Here's how the part is built. I have some questions about the finished solid (model axes, mm). Coordinates: 2 decimals unless noted, no trailing zeros. Write each loop counter-clockwise with the first axis right and the second up, starting at its lowest first coordinate (ties: lowest second). Pieces come first, ordered by that corner, then holes.
(1) Imagine slicing it at B-B, the plane y = 0.4. State how many separate pieces and enclosed holes the cut face has, plus the area to 3 significant figures.
(2) Imagine slicing it at A-A, the plane z = 63.56. List the corners of the cut face in (x, y) for me.
(3) For pin 1 Ø1 at (x, y) = (36, 0.5) entering from -Z, with a flat end and sliding along its axis, tell me the tip position at first contact or that it passes through.
(4) Imagine slicing it at C-C, the plane x = 66.72. List the corners of the cut face in (y, z) for me (3 decimals), plus the area to 3 significant figures.
(5) Imagine slicing it at D-D, the plane x = 52.22. List the corners of the cut face in (y, z) for me, plus the area to 3 significant figures.
(6) Thinking about a two-plate mould opening in Z: for faces 1 (the flat face through (-3, 1, 48)), 2 (the cylindrical face through (64.963, 0.986, 68.005)), 3 (the cylindrical face through (76.17, 0.99, 72.1)), which applies, released by +Z, released by -Z, zero draft, split by the parting line, or undercut?
(7) Please list where these lines run through material, in increasing order: probe 1 along X at (y, z) = (1.3, 31.49); probe 2 along Z at (x, y) = (23.5, 1.15); probe 3 along Z at (x, y) = (24, 1.4).
```python
from build123d import *

# Parameters (mm, degrees)
CROQUIS1_R              = 1.8
CROQUIS1_R_2            = 1.5
SALIENTE_EXTRUIR1_DEPTH = 2


with BuildPart() as part:
    # Croquis1 → Saliente-Extruir1 (new body)
    with BuildSketch(Plane(origin=(0, 0, 0), x_dir=(1, 0, 0), z_dir=(0, 1, 0))):
        with BuildLine():
            Line((0.952532669, 2.844763877), (74.672532669, -21.839431846))
            ThreePointArc((74.672532669, -21.839431846), (76.154912525, -22.931711487), (76.72, -24.684195722))
            Line((76.72, -24.684195722), (76.72, -70.365804278))
            ThreePointArc((76.72, -70.365804278), (76.154912525, -72.118288513), (74.672532669, -73.210568154))
            Line((74.672532669, -73.210568154), (0.952532669, -97.894763877))
            ThreePointArc((0.952532669, -97.894763877), (-1.752484236, -97.484912525), (-3, -95.05))
            Line((-3, -95.05), (-3, 0))
            ThreePointArc((-3, 0), (-1.752484236, 2.434912525), (0.952532669, 2.844763877))
        make_face()
        with Locations(Location((25, -26.675, 0), (0, 0, 270))):
            Circle(CROQUIS1_R, mode=Mode.SUBTRACT)
        with Locations(Location((25, -68.395, 0), (0, 0, 270))):
            Circle(CROQUIS1_R, mode=Mode.SUBTRACT)
        with Locations(Location((66.72, -26.675, 0), (0, 0, 270))):
            Circle(CROQUIS1_R, mode=Mode.SUBTRACT)
        with Locations(Location((66.72, -68.395, 0), (0, 0, 270))):
            Circle(CROQUIS1_R, mode=Mode.SUBTRACT)
        with Locations(Location((0, 0, 0), (0, 0, 270))):
            Circle(CROQUIS1_R_2, mode=Mode.SUBTRACT)
        with Locations(Location((0, -95.05, 0), (0, 0, 270))):
            Circle(CROQUIS1_R_2, mode=Mode.SUBTRACT)
        with Locations(Location((52.22, -31.49, 0), (0, 0, 270))):
            Circle(CROQUIS1_R_2, mode=Mode.SUBTRACT)
        with Locations(Location((52.22, -63.56, 0), (0, 0, 270))):
            Circle(CROQUIS1_R_2, mode=Mode.SUBTRACT)
    extrude(amount=SALIENTE_EXTRUIR1_DEPTH)


solid = part.part
```
Recorded:
1. separate pieces: 1
1. enclosed holes: 8
1. area: 6,040 mm2
2. outline: (-3, 0) - (50.72, 0) - (50.72, 2) - (-3, 2) - close; (53.72, 0) - (76.72, 0) - (76.72, 2) - (53.72, 2) - close
3. pin 1: stops at z = 8.72
4. outline: (0, 19.177) - (2, 19.177) - (2, 24.875) - (0, 24.875) - close; (0, 28.475) - (2, 28.475) - (2, 66.595) - (0, 66.595) - close; (0, 70.195) - (2, 70.195) - (2, 75.873) - (0, 75.873) - close
4. area: 99.0 mm2
5. outline: (0, 14.32) - (2, 14.32) - (2, 29.99) - (0, 29.99) - close; (0, 32.99) - (2, 32.99) - (2, 62.06) - (0, 62.06) - close; (0, 65.06) - (2, 65.06) - (2, 80.73) - (0, 80.73) - close
5. area: 121 mm2
6. face 1: zero draft
6. face 2: undercut
6. face 3: released by +Z
7. probe 1: x = -3 to 50.72, 53.72 to 76.72
7. probe 2: z = 4.7 to 25.68, 27.67 to 67.4, 69.39 to 90.35
7. probe 3: z = 4.87 to 25.18, 28.17 to 66.9, 69.89 to 90.18
